Part model, mm, in its own coordinate system. A direction names the side the tool comes from. Give positions to 0.01 mm unless a question says otherwise; leave off trailing zeros. Loops run counter-clockwise (first coordinate to the right, second up) from the corner with the lowest first, then second, coordinate; pieces in that order, holes last. Notation, with made-up numbers: (37, 56.5) -> (89, 56.5) arc R29 ccw to (89, 84.5) -> close; hole circle Ø2 at (65.25, 43.5). An arc over 180 degrees is marked (long way). One line per question, with ' | ' between items.
```python
from build123d import *

# Parameters (mm, degrees)
FILLET1_R                  = 1
M16X2_0_TAPPED_HOLE1_D     = 14
M16X2_0_TAPPED_HOLE1_DEPTH = 38
M16X2_0_TAPPED_HOLE1_TIP   = 4.206024333


with BuildPart() as part:
    # Sketch1 → Revolve1 (revolve)
    with BuildSketch(Plane.XY):
        with BuildLine():
            Line((89, 65), (51, 65))
            Line((51, 65), (51, 58))
            Line((51, 58), (41.3, 58))
            Line((41.3, 58), (41.3, 65))
            Line((41.3, 65), (0, 65))
            Line((0, 65), (0, 55))
            Line((0, 55), (-5, 55))
            Line((-5, 55), (-5, 59.5))
            Line((-5, 59.5), (-15, 59.5))
            ThreePointArc((-15, 59.5), (-16.414213562, 60.085786438), (-17, 61.5))
            Line((-17, 61.5), (-17, 109.5))
            ThreePointArc((-17, 109.5), (-11.142135624, 123.642135624), (3, 129.5))
            Line((3, 129.5), (7.686032459, 129.5))
            Line((7.686032459, 129.5), (7.686032459, 217))
            Line((7.686032459, 217), (17.686032459, 217))
            Line((17.686032459, 217), (17.686032459, 77))
            Line((17.686032459, 77), (89, 77))
            Line((89, 77), (89, 65))
        make_face()
    revolve(axis=Axis((131.481481481, 0, 0), (-1, 0, 0)))

    # Fillet1
    fillet1_edges = [part.edges().sort_by_distance(p)[0] for p in [
        (41.3, -65, 0),
        (51, -65, 0),
    ]]
    fillet(fillet1_edges, radius=FILLET1_R)

    # M16x2.0 Tapped Hole1
    with Locations(Plane.ZY.offset(-7.686032459)):
        with Locations((0, 197), (0, -197), (162, -112.093710796), (-162, -112.093710796), (-162, 112.093710796), (162, 112.093710796)):
            Hole(M16X2_0_TAPPED_HOLE1_D / 2, depth=M16X2_0_TAPPED_HOLE1_DEPTH)
            with Locations((0, 0, -(M16X2_0_TAPPED_HOLE1_DEPTH + M16X2_0_TAPPED_HOLE1_TIP / 2))):  # 118° drill point
                Cone(0, M16X2_0_TAPPED_HOLE1_D / 2, M16X2_0_TAPPED_HOLE1_TIP, mode=Mode.SUBTRACT)


solid = part.part
```
1) Saw through at B-B (y = -197). Give the cut face in (x, z).
Found:
outline: (7.69, -90.99) -> (17.69, -90.99) -> (17.69, -7) -> (7.69, -7) -> close; (7.69, 7) -> (17.69, 7) -> (17.69, 90.99) -> (7.69, 90.99) -> close
2) Drill centre lines: line 1 (Y direction, x = 11.25, z = 0); line 2 (Z direction, x = 45, y = 0); line 3 (Y direction, x = 12.75, z = -162). Where is each one in solid material? Low to high.
Found:
line 1: -217 to -204, -190 to -65, 65 to 190, 204 to 217 | line 2: -77 to -58, 58 to 77 | line 3: -144.38 to -119.09, -105.09 to 105.09, 119.09 to 144.38
3) Tool access for faces 1 (the flat face through (89, -52, 40)), 2 (the cylindrical face through (12.76, -114.77, 155.53)), 3 (the cylindrical face through (5.376, -102.767, 78.799)), 4 (the cylindrical face through (46.08, 26.76, 51.46)), 5 (the flat face through (0, -53.3, -14.7)): list every direction of +Z, -Z, +X, -X, +Y, -Y with a clear straight run to the whole face (end or side of a thin tool).
Found:
face 1: +Z, -Z, +X, +Y, -Y | face 2: +X, -X | face 3: -X | face 4: +X | face 5: none
4) Saw through at A-A (z = -162). Give the cut face in (x, y).
Found:
outline: (7.69, -144.38) -> (17.69, -144.38) -> (17.69, -119.09) -> (7.69, -119.09) -> close; (7.69, -105.09) -> (17.69, -105.09) -> (17.69, 105.09) -> (7.69, 105.09) -> close; (7.69, 119.09) -> (17.69, 119.09) -> (17.69, 144.38) -> (7.69, 144.38) -> close
5) Saw through at D-D (z = 0). State how many separate pieces and enclosed holes the cut face has, and give its area (3 significant figures).
Found:
separate pieces: 4 | enclosed holes: 0 | area: 7,850 mm2
6) Pin check, flat tips, straight feed: P1, Ø22.5, axis at y = 112.09, z = 162, coming from the -X side; P2, Ø1, axis at y = -152.5, z = 90, coming from the +X side; P3, Ø1, axis at x = 57.5, y = 63, coming from the +Z side (3 decimals). Stop position of each tip, or through.
Found:
P1: x = 7.69 | P2: x = 17.69 | P3: z = 44.975
7) Saw through at C-C (x = 77). Give the cut face in (y, z), and give its area (3 significant figures).
Found:
outline: circle Ø154 at (0, 0); hole circle Ø130 at (0, 0) | area: 5,350 mm2
8) Pull direction X, two halves, no side cores. Call faces 6 (the cylindrical face through (-2.535, -11.923, 53.692)), 7 (the flat face through (51, -33, -48)), 8 (the flat face through (41.3, 33, -48)): pulls with the +X half, pulls with the -X half, needs draft (parallel to the pull), parting line crosses it, or undercut.
Found:
face 6: needs draft | face 7: pulls with the +X half | face 8: undercut
